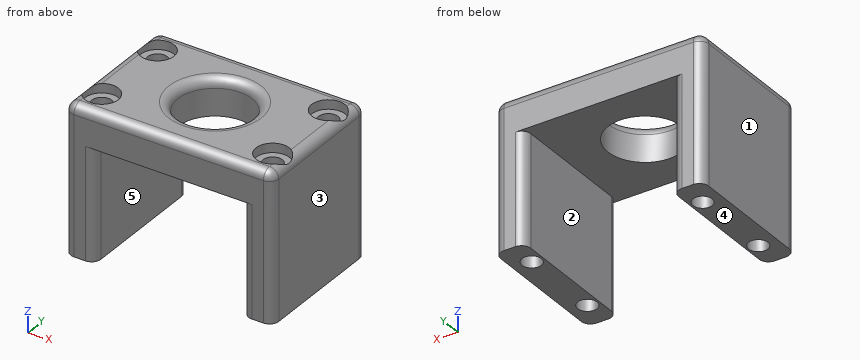
Autodesk Inventor part; units mm, degrees
ref_plane "Arbeitsebene2" through (-7.2804, -7.2804, 24.15) normal (0, 0, -1) x (-0.0257355, 0.9996688, 0)
ref_plane "YZ Plane" through (0, 0, 0) normal (1, 0, 0) x (0, 1, 0)
ref_plane "XZ Plane" through (0, 0, 0) normal (0, 1, 0) x (-1, 0, 0)
sketch "Skizze1" plane through (0, 0, 0) normal (0, 0, 1) x (1, 0, 0)
  circle A0 centre (0, 0) radius 8 construction
  line L0 (-30, -17.5) -> (30, -17.5) construction
  line L1 (30, -17.5) -> (30, 17.5) construction
  line L2 (30, 17.5) -> (-30, 17.5) construction
  line L3 (-30, 17.5) -> (-30, -17.5) construction
  circle A1 centre (0, 0) radius 9 construction
  circle A2 centre (0, 0) radius 14 construction
  line L4 (-15, -15) -> (15, -15)
  line L5 (15, 15) -> (-15, 15)
  line L6 (-15, -15) -> (15, 15) construction
  line L7 (15, -15) -> (-15, 15) construction
  line L8 (-22.5, -15) -> (22.5, -15)
  line L9 (22.5, -15) -> (22.5, 15)
  line L10 (22.5, 15) -> (-22.5, 15)
  line L11 (-22.5, 15) -> (-22.5, -15)
  line L12 (-22.5, -15) -> (22.5, 15) construction
  line L13 (22.5, -15) -> (-22.5, 15) construction
  circle A3 centre (0, 0) radius 8
  point P0 (0, 0)
extrude "Extrusion1" add sketch "Skizze1" along normal blind 32
ref_plane "Arbeitsebene1" through (0, 0, 0) normal (0, 0, 1) x (1, 0, 0)
sketch "Skizze2" plane through (0, 0, 0) normal (0, 0, 1) x (1, 0, 0)
  circle A0 centre (0, 0) radius 13.8 construction
  circle A1 centre (0, 0) radius 14 construction
  line L0 (22.5, 15) -> (-22.5, 15) construction
  line L1 (22.5, -15) -> (22.5, 15) construction
  line L2 (-22.5, -15) -> (22.5, -15) construction
  line L3 (-22.5, 15) -> (-22.5, -15) construction
  line L4 (-22.5, -15) -> (22.5, -15)
  line L5 (-16, 15) -> (16, 15)
  line L6 (16, 15) -> (16, -15)
  line L7 (16, -15) -> (-16, -15)
  line L8 (-16, -15) -> (-16, 15)
  line L9 (-16, 15) -> (16, -15) construction
  line L10 (16, 15) -> (-16, -15) construction
  point P0 (0, 0)
  dimension "d5" = 32
ref_plane "Arbeitsebene2" through (-7.2804, -7.2804, 24.15) normal (0, 0, -1) x (-0.0257355, 0.9996688, 0)
extrude "Extrusion2" cut sketch "Skizze2" along normal up to surface (24.15 mm away)
sketch "Skizze3" plane through (0, 0, 32) normal (0, 0, 1) x (1, 0, 0)
  circle A0 centre (0, 0) radius 8 construction
  line L0 (-22.5, -15) -> (22.5, -15) construction
  line L1 (22.5, -15) -> (22.5, 15) construction
  line L2 (22.5, 15) -> (-22.5, 15) construction
  line L3 (-22.5, 15) -> (-22.5, -15) construction
  line L4 (16, -15) -> (16, 15) construction
  line L5 (-16, 15) -> (-16, -15) construction
  line L6 (22.5, -11.8361) -> (18.5, -11.8361) construction
  line L7 (16, -15) -> (22.5, -15) construction
  line L8 (18.5, -15) -> (18.5, -9) construction
  line L9 (22.5, 15) -> (-22.5, 15) construction
  line L10 (18.5, 15) -> (18.5, 9) construction
  line L11 (-22.5, 15) -> (-22.5, -15) construction
  line L12 (-22.5, -9) -> (-18.4855, -9) construction
  line L13 (-22.5, 9) -> (-18.4855, 9) construction
  point P0 (0, 0)
  dimension "d9" = 4
  dimension "d10" = 6
  dimension "d11" = 6
hole "Bohrung1" at (18.5, -9, 32) at (18.5, 9, 32) at (-18.4855, -9, 32) at (-18.4855, 9, 32) direction (0, 0, -1) diameter 4.2 end through all counterbore diameter 7.2 counterbore depth 2
fillet "Rundung1" radius 2 4 edges at (0, -15, 32) (22.5, 0, 32) (0, 15, 32) (-22.5, 0, 32)
fillet "Rundung2" radius 2 1 edges at (-8, 0, 32)
fillet "Rundung3" radius 2 12 edges at (21.9142, 14.4142, 31.4142) (22.5, 15, 15) (16, 15, 12.075) (-16, 15, 12.075) (-21.9142, 14.4142, 31.4142) (-22.5, 15, 15) (21.9142, -14.4142, 31.4142) (22.5, -15, 15) (-21.9142, -14.4142, 31.4142) (-22.5, -15, 15) (-16, -15, 12.075) (16, -15, 12.075)
properties part number "Upper_bearing_support_outside"
Geometry check sheet. Reference: the model listing, model coordinates, mm. Face numbers are marked on the shaded views. A direction names the side the tool comes from. Give positions to 0.01 mm unless a question says otherwise; leave off trailing zeros. Order: outer loops, then holes, each group sorted by start corner. A loop starts at its lowest first (then second) coordinate and runs counter-clockwise, first axis right, second up. Notation, with made-up numbers: (40.5, 56.25) - (70.5, 56.25) arc R20 cw to (70.5, 67.25) - close; hole circle Ø3 at (-36.5, -28). An arc over 180 degrees is marked (long way). Answer in a Markdown table with one row per item. Add a question column.
Q1. Cross-section at A-A, the plane y = 0. Enter the section's corners in (x, z), then the cut area to 3 significant figures.
Q2. Tool access check on the marked faces 4 and 5. Record the directions out of +Z, -Z, +X, -X, +Y, -Y that give a thin tool (end or side, any length) a straight path to the whole face; none if there is none.
Q3. Cross-section at C-C, the plane z = 20. Enter the section's corners in (x, y).
Q4. Material ranges on probe 1 along X at (y, z) = (9, 6); probe 2 along Y at (x, z) = (18.5, 9.25); probe 3 along X at (y, z) = (-4.25, 13), recorded low to high. Write a range as from..to.
Q5. Mould release check, pull along X, two halves, no side actions. Record for the marked faces 1, 2 and 3: pulls with the +X half, pulls with the -X half, needs draft (parallel to the pull), parting line crosses it, or undercut.
Q6. Gauge pin test, flat ends, axial feed: pin 1 (1 mm diameter, centred on x = 7, y = -11.5, fed in from -Z); pin 2 (6 mm diameter, centred on x = 18.5, y = -9, fed in from +Z). Record the tip position at first contact, or that the pin passes through.
Q7. Cross-section at B-B, the plane x = 0. Enter the section's corners in (y, z).
Q8. Cross-section at D-D, the plane x = 13.5. Enter the section's corners in (y, z), then the cut area to 3 significant figures.
Check values:
| question | item | result |
|---|---|---|
| 1 | outline | (-22.5, 0) - (-16, 0) - (-16, 24.15) - (-8, 24.15) - (-8, 30) arc R2 ccw to (-10, 32) - (-20.5, 32) arc R2 ccw to (-22.5, 30) - close; (8, 24.15) - (16, 24.15) - (16, 0) - (22.5, 0) - (22.5, 30) arc R2 ccw to (20.5, 32) - (10, 32) arc R2 ccw to (8, 30) - close |
| 1 | area | 538 mm^2 |
| 2 | face 4 | -Z, +X, -X, +Y, -Y |
| 2 | face 5 | -Z, +Y, -Y |
| 3 | outline | (-22.5, -13) arc R2 ccw to (-20.5, -15) - (-18, -15) arc R2 ccw to (-16, -13) - (-16, 13) arc R2 ccw to (-18, 15) - (-20.5, 15) arc R2 ccw to (-22.5, 13) - close; (16, -13) arc R2 ccw to (18, -15) - (20.5, -15) arc R2 ccw to (22.5, -13) - (22.5, 13) arc R2 ccw to (20.5, 15) - (18, 15) arc R2 ccw to (16, 13) - close; hole circle Ø4.2 at (-18.49, -9); hole circle Ø4.2 at (-18.49, 9); hole circle Ø4.2 at (18.5, -9); hole circle Ø4.2 at (18.5, 9) |
| 4 | probe 1 | x = -22.5..-20.59, -16.39..-16, 16..16.4, 20.6..22.5 |
| 4 | probe 2 | y = -15..-11.1, -6.9..6.9, 11.1..15 |
| 4 | probe 3 | x = -22.5..-16, 16..22.5 |
| 5 | face 1 | pulls with the -X half |
| 5 | face 2 | undercut |
| 5 | face 3 | pulls with the +X half |
| 6 | pin 1 | stops at z = 24.15 |
| 6 | pin 2 | stops at z = 30 |
| 7 | outline | (-15, 24.15) - (-8, 24.15) - (-8, 30) arc R2 ccw to (-10, 32) - (-13, 32) arc R2 ccw to (-15, 30) - close; (8, 24.15) - (15, 24.15) - (15, 30) arc R2 ccw to (13, 32) - (10, 32) arc R2 ccw to (8, 30) - close |
| 8 | outline | (-15, 24.15) - (15, 24.15) - (15, 30) arc R2 ccw to (13, 32) - (-13, 32) arc R2 ccw to (-15, 30) - close |
| 8 | area | 234 mm^2 |
